Input: part model. Units: mm. Frame: model coordinates. Round coordinates to 2 decimals unless told otherwise and drop trailing zeros. Loops run counter-clockwise (first coordinate to the right, second up) from the corner with the lowest first, then second, coordinate; pieces in that order, holes last.
(1) Cut plane B-B, the plane x = 4. Output: boundary loops of the cut face in (y, z), and give its area (3 significant figures).
(2) Cut plane C-C, the plane y = 0.7. Give the number of separate pieces and of enclosed holes in the cut face, and give its area (3 significant figures).
(3) Cut plane A-A, the plane x = -14. Output: boundary loops of the cut face in (y, z), and give its area (3 significant figures).
(4) Line query: line 1 (Z direction, x = -8, y = 0.95); line 2 (Z direction, x = 17.5, y = 3.3); line 3 (X direction, y = 3.8, z = -6). Output: solid intervals per line, ascending.
(5) Draft query along X for faces 1 (the face through (0, 2, -15)), 2 (the face through (-18.485, 2.028, 5.583)). Return one class per face: released by +X, released by -X, zero draft, split by the parting line, or undercut.
(6) First-contact query: pin 1 Ø1.8 at (x, z) = (39.725, 0) entering from +Y (3 decimals); pin 2 Ø13 at (x, z) = (30.225, 0) entering from -Y; pin 3 Ø1.5 at (y, z) = (2, 3.5) entering from +X. Flat tips, straight axial feed; report the tip coordinate or a pass-through.
from build123d import *

# Parameters (mm, degrees)
SKETCH_1_R          = 5
SKETCH_1_R_2        = 1.5
SKETCH_1_R_3        = 1.25
EXTRUDE_1_DEPTH     = 4
CUT_EXTRUDE_1_DEPTH = 10
FILLET_1_R          = 2.5
FILLET_2_R          = 3
CUT_EXTRUDE_2_DEPTH = 10
CHAMFER_1_SIZE      = 1.5


with BuildPart() as part:
    # 草图1 → 凸台-拉伸1 (new body)
    with BuildSketch(Plane(origin=(0, 0, 0), x_dir=(1, 0, 0), z_dir=(0, 1, 0))):
        with BuildLine():
            Line((-30.225, 15), (30.225, 15))
            ThreePointArc((30.225, 15), (45.225, 0), (30.225, -15))
            Line((30.225, -15), (-30.225, -15))
            ThreePointArc((-30.225, -15), (-45.225, 0), (-30.225, 15))
        make_face()
        with Locations(Location((-30.225, 0, 0), (0, 0, 270))):
            Circle(SKETCH_1_R, mode=Mode.SUBTRACT)
        with Locations(Location((30.225, 0, 0), (0, 0, 90))):
            Circle(SKETCH_1_R, mode=Mode.SUBTRACT)
        with Locations(Location((-30.225, 9.5, 0), (0, 0, 270))):
            Circle(SKETCH_1_R_2, mode=Mode.SUBTRACT)
        with Locations(Location((-30.225, -9.5, 0), (0, 0, 90))):
            Circle(SKETCH_1_R_2, mode=Mode.SUBTRACT)
        with Locations(Location((-38.225, 0, 0), (0, 0, 270))):
            Circle(SKETCH_1_R_2, mode=Mode.SUBTRACT)
        with Locations(Location((-22.225, 0, 0), (0, 0, 90))):
            Circle(SKETCH_1_R_2, mode=Mode.SUBTRACT)
        with Locations(Location((30.225, 8, 0), (0, 0, 270))):
            Circle(SKETCH_1_R_2, mode=Mode.SUBTRACT)
        with Locations(Location((20.725, 0, 0), (0, 0, 270))):
            Circle(SKETCH_1_R_2, mode=Mode.SUBTRACT)
        with Locations(Location((39.725, 0, 0), (0, 0, 90))):
            Circle(SKETCH_1_R_2, mode=Mode.SUBTRACT)
        with Locations(Location((30.225, -8, 0), (0, 0, 90))):
            Circle(SKETCH_1_R_2, mode=Mode.SUBTRACT)
        with Locations(Location((0, -1, 0), (0, 0, 270))):
            Circle(SKETCH_1_R_3, mode=Mode.SUBTRACT)
    extrude(amount=EXTRUDE_1_DEPTH)

    # 草图2 → 切除-拉伸1 (cut)
    with BuildSketch(Plane(origin=(0, 4, 0), x_dir=(1, 0, 0), z_dir=(0, 1, 0))):
        with BuildLine():
            Line((-3.092329219, -2), (-17.379767421, -2))
            ThreePointArc((-17.379767421, -2), (-19.996946351, -8.02414597), (-25.225, -12))
            Line((-25.225, -12), (25.225, -12))
            ThreePointArc((25.225, -12), (19.996946351, -8.02414597), (17.379767421, -2))
            Line((17.379767421, -2), (3.092329219, -2))
            ThreePointArc((3.092329219, -2), (0, -4.25), (-3.092329219, -2))
        make_face()
        with BuildLine():
            Line((-17.379767421, 2), (-1.25, 2))
            ThreePointArc((-1.25, 2), (0, 2.25), (1.25, 2))
            Line((1.25, 2), (17.379767421, 2))
            ThreePointArc((17.379767421, 2), (19.996946351, 8.02414597), (25.225, 12))
            Line((25.225, 12), (-25.225, 12))
            ThreePointArc((-25.225, 12), (-19.996946351, 8.02414597), (-17.379767421, 2))
        make_face()
    extrude(amount=-CUT_EXTRUDE_1_DEPTH, mode=Mode.SUBTRACT)

    # 圆角1
    fillet_1_edges = [part.edges().sort_by_distance(p)[0] for p in [
        (-25.225, 2, -12),
        (25.225, 2, -12),
        (17.379767421, 2, 2),
        (-17.379767421, 2, 2),
    ]]
    fillet(fillet_1_edges, radius=FILLET_1_R)

    # 圆角2
    fillet_2_edges = [part.edges().sort_by_distance(p)[0] for p in [
        (1.25, 2, -2),
        (-1.25, 2, -2),
        (-17.379767421, 2, -2),
        (17.379767421, 2, -2),
        (-3.092329219, 2, 2),
        (3.092329219, 2, 2),
        (25.225, 2, 12),
        (-25.225, 2, 12),
    ]]
    fillet(fillet_2_edges, radius=FILLET_2_R)

    # 草图3 → 切除-拉伸2 (cut)
    with BuildSketch(Plane(origin=(0, 4, 0), x_dir=(1, 0, 0), z_dir=(0, 1, 0))):
        with BuildLine():
            ThreePointArc((-34.867857143, 5.890150894), (-34.368939643, 10.103354108), (-38.582142857, 10.602271609))
            ThreePointArc((-38.582142857, 10.602271609), (-39.770941546, 9.545941546), (-40.827271609, 8.357142857))
            ThreePointArc((-40.827271609, 8.357142857), (-40.328354108, 4.143939643), (-36.115150894, 4.642857143))
            ThreePointArc((-36.115150894, 4.642857143), (-35.528300859, 5.303300859), (-34.867857143, 5.890150894))
        make_face()
        with BuildLine():
            ThreePointArc((-40.827271609, -8.357142857), (-39.770941546, -9.545941546), (-38.582142857, -10.602271609))
            ThreePointArc((-38.582142857, -10.602271609), (-34.368939643, -10.103354108), (-34.867857143, -5.890150894))
            ThreePointArc((-34.867857143, -5.890150894), (-35.528300859, -5.303300859), (-36.115150894, -4.642857143))
            ThreePointArc((-36.115150894, -4.642857143), (-40.328354108, -4.143939643), (-40.827271609, -8.357142857))
        make_face()
        with BuildLine():
            ThreePointArc((38.582142857, -10.602271609), (39.770941546, -9.545941546), (40.827271609, -8.357142857))
            ThreePointArc((40.827271609, -8.357142857), (40.328354108, -4.143939643), (36.115150894, -4.642857143))
            ThreePointArc((36.115150894, -4.642857143), (35.528300859, -5.303300859), (34.867857143, -5.890150894))
            ThreePointArc((34.867857143, -5.890150894), (34.368939643, -10.103354108), (38.582142857, -10.602271609))
        make_face()
        with BuildLine():
            ThreePointArc((40.827271609, 8.357142857), (39.770941546, 9.545941546), (38.582142857, 10.602271609))
            ThreePointArc((38.582142857, 10.602271609), (34.368939643, 10.103354108), (34.867857143, 5.890150894))
            ThreePointArc((34.867857143, 5.890150894), (35.528300859, 5.303300859), (36.115150894, 4.642857143))
            ThreePointArc((36.115150894, 4.642857143), (40.328354108, 4.143939643), (40.827271609, 8.357142857))
        make_face()
    extrude(amount=-CUT_EXTRUDE_2_DEPTH, mode=Mode.SUBTRACT)

    # 倒角1
    chamfer_1_edges = [part.edges().sort_by_distance(p)[0] for p in [
        (0, 0, -0.25),
    ]]
    chamfer(chamfer_1_edges, length=CHAMFER_1_SIZE)


solid = part.part
Reported:
1. outline: (0, -15) - (4, -15) - (4, -12) - (0, -12) - close; (0, -2) - (4, -2) - (4, 2.11) - (0, 2.11) - close; (0, 12) - (4, 12) - (4, 15) - (0, 15) - close
1. area: 40.4 mm2
2. separate pieces: 1
2. enclosed holes: 17
2. area: 1,380 mm2
3. outline: (0, -15) - (4, -15) - (4, -12) - (0, -12) - close; (0, -2) - (4, -2) - (4, 2) - (0, 2) - close; (0, 12) - (4, 12) - (4, 15) - (0, 15) - close
3. area: 40.0 mm2
4. line 1: z = -15 to -12, -2 to 2, 12 to 15
4. line 2: z = -15 to -12, -3.3 to 3.16, 11.96 to 15
4. line 3: x = -43.97 to -41.43, -34.74 to -18.69, 18.69 to 34.74, 41.43 to 43.97
5. face 1: zero draft
5. face 2: undercut
6. pin 1: passes through
6. pin 2: stops at y = 0
6. pin 3: stops at x = 44.97
